from build123d import *

# Parameters (mm, degrees)
SKETCH1_W               = 63.85
SKETCH1_H               = 96.52
BOSS_EXTRUDE1_DEPTH     = 3
SKETCH5_W               = 8
SKETCH5_H               = 3
CUT_EXTRUDE3_DEPTH      = 3
CUT_EXTRUDE6_DEPTH      = 1
CUT_EXTRUDE6_DEPTH_BACK = 3
SKETCH21_W              = 0.5
SKETCH21_H              = 3
CUT_EXTRUDE11_DEPTH     = 3
FILLET17_R              = 1
FILLET18_R              = 1
SKETCH22_W              = 96.52
SKETCH22_H              = 3
CUT_EXTRUDE12_DEPTH     = 17.25


with BuildPart() as part:
    # Sketch1 → Boss-Extrude1 (new body)
    with BuildSketch(Plane(origin=(0, 0, 0), x_dir=(1, 0, 0), z_dir=(0, 1, 0))):
        Rectangle(SKETCH1_W, SKETCH1_H)
    extrude(amount=BOSS_EXTRUDE1_DEPTH)

    # Sketch5 → Cut-Extrude3 (cut)
    with BuildSketch(Plane.XY.offset(48.26)):
        with Locations((24.925, 1.5)):
            Rectangle(SKETCH5_W, SKETCH5_H)
    cut_extrude3 = extrude(amount=-CUT_EXTRUDE3_DEPTH, mode=Mode.SUBTRACT)

    # Sketch20 → Cut-Extrude6 (cut, two sides)
    with BuildSketch(Plane.XY.offset(48.26)) as cut_extrude6_sk:
        Polygon((31.425, 139.841988316), (31.425, 3), (31.425, 0), (31.425, -136.841988316), (305.108976632, -136.841988316), (305.108976632, 139.841988316), align=None)
    extrude(amount=CUT_EXTRUDE6_DEPTH, mode=Mode.SUBTRACT)
    extrude(cut_extrude6_sk.sketch, amount=-CUT_EXTRUDE6_DEPTH_BACK, mode=Mode.SUBTRACT)

    # Mirror1: Cut-Extrude3 across plane
    add(cut_extrude3.mirror(Plane.XY), mode=Mode.SUBTRACT)

    # Sketch21 → Cut-Extrude11 (cut)
    with BuildSketch(Plane(origin=(0, 0, -48.26), x_dir=(-1, 0, 0), z_dir=(0, 0, -1))):
        with Locations((-31.675, 1.5)):
            Rectangle(SKETCH21_W, SKETCH21_H)
    extrude(amount=-CUT_EXTRUDE11_DEPTH, mode=Mode.SUBTRACT)

    # Fillet17
    fillet17_edges = [part.edges().sort_by_distance(p)[0] for p in [
        (28.925, 3, 46.76),
        (28.925, 0, 46.76),
        (31.425, 3, 46.76),
        (31.425, 0, 46.76),
    ]]
    fillet(fillet17_edges, radius=FILLET17_R)

    # Fillet18
    fillet18_edges = [part.edges().sort_by_distance(p)[0] for p in [
        (28.925, 3, -46.76),
        (28.925, 0, -46.76),
        (31.425, 3, -46.76),
        (31.425, 0, -46.76),
    ]]
    fillet(fillet18_edges, radius=FILLET18_R)

    # Sketch22 → Cut-Extrude12 (cut)
    with BuildSketch(Plane.ZY.offset(31.925)):
        with Locations((0, 1.5)):
            Rectangle(SKETCH22_W, SKETCH22_H)
    extrude(amount=-CUT_EXTRUDE12_DEPTH, mode=Mode.SUBTRACT)


solid = part.part
Check sheet for the modelled part. Datum: model origin and axes. Units: mm. Give positions to 0.01 mm unless a question says otherwise; leave off trailing zeros. Use one line per item in the form item = value. Start each with the question number.
1. Thickness scan on line 1 along Z through (x, y) = (26, 0.15). Record the ranges inside material, lowest first. Write a range as from..to.
2. Mould release check, pull along X, two halves, no side actions. Record for faces 1 (the flat face through (20.925, 1, -47)), 2 (the flat face through (3, 1, 48.26)), 3 (the flat face through (20.925, 1, 47)), 4 (the flat face through (31.925, 1, 1)): pulls with the +X half, pulls with the -X half, needs draft (parallel to the pull), parting line crosses it, or undercut.
3. Go/stop test with flat-tipped pins: P1, Ø3, axis at x = 16, z = 20.5, coming from the -Y side; P2, Ø0.5, axis at y = 1.5, z = -46.5, coming from the +X side (3 decimals); P3, Ø0.9, axis at x = 25.5, y = 1.5, coming from the +Z side; P4, Ø1.5, axis at x = 23.5, y = 1, coming from the -Z side. Record where each tip stops, or that it passes through.
Conclusion:
q1.line_1 = -45.26..45.26
q2.face_1 = undercut
q2.face_2 = needs draft
q2.face_3 = undercut
q2.face_4 = pulls with the +X half
q3.P1 = 0
q3.P2 = 31.425
q3.P3 = 45.26
q3.P4 = -45.26
